Model file for the job. Use its own axes, mm. A direction names the side the tool comes from. Coordinates: 2 decimals unless noted, no trailing zeros. Write each loop counter-clockwise with the first axis right and the second up, starting at its lowest first coordinate (ties: lowest second). Pieces come first, ordered by that corner, then holes. Notation, with made-up numbers: M -37,-32.5 L -23,-32.5 A28 cw -23,-4.5 Z; hole C -26,47 d9. An arc over 180 degrees is marked long. Answer in a Markdown table with one row per item. Add a question column.
```python
from build123d import *

# Parameters (mm, degrees)
SKETCH_1_W          = 26
SKETCH_1_H          = 23.5
SKETCH_1_W_2        = 24
SKETCH_1_H_2        = 21.5
EXTRUDE_1_DEPTH     = 10
SKETCH_2_W          = 12.504676962
SKETCH_2_H          = 3.66933463
CUT_EXTRUDE_1_DEPTH = 1
EXTRUDE_2_DEPTH     = 2.3
SKETCH_5_W          = 26
SKETCH_5_H          = 23.5
EXTRUDE_3_DEPTH     = 1
CUT_EXTRUDE_2_REACH = 38.168
SKETCH_6_W          = 24.2
SKETCH_6_H          = 21.7
SKETCH_6_W_2        = 24
SKETCH_6_H_2        = 21.5
SKETCH_7_W          = 22.2
SKETCH_7_H          = 1
SKETCH_7_W_2        = 1
SKETCH_7_H_2        = 19.7
SKETCH_7_W_3        = 6.19724131
SKETCH_7_H_3        = 1.03
SKETCH_7_W_4        = 6.2
EXTRUDE_4_DEPTH     = 5.75
FILLET_1_R          = 0.95


with BuildPart() as part:
    # 草图1 → 凸台-拉伸1 (new body)
    with BuildSketch(Plane(origin=(0, 0, 0), x_dir=(1, 0, 0), z_dir=(0, 1, 0))):
        with Locations((12, 10.75)):
            Rectangle(SKETCH_1_W, SKETCH_1_H)
        with Locations((12, 10.75)):
            Rectangle(SKETCH_1_W_2, SKETCH_1_H_2, mode=Mode.SUBTRACT)
    extrude(amount=EXTRUDE_1_DEPTH)

    # 草图2 → 切除-拉伸1 (cut)
    with BuildSketch(Plane.ZY.offset(1)):
        with Locations((-10.334237592, 1.834667315)):
            Rectangle(SKETCH_2_W, SKETCH_2_H)
    extrude(amount=-CUT_EXTRUDE_1_DEPTH, mode=Mode.SUBTRACT)

    # 草图3 → 凸台-拉伸2 (add)
    with BuildSketch(Plane.XZ):
        Polygon((-1, -4.081899111), (-1, 1), (25, 1), (25, -22.5), (-1, -22.5), (-1, -16.586576073), (0, -16.586576073), (0, -21.5), (24, -21.5), (24, 0), (0, 0), (0, -4.081899111), align=None)
    extrude(amount=EXTRUDE_2_DEPTH)

    # 草图5 → 凸台-拉伸3 (add)
    with BuildSketch(Plane.XZ.offset(2.3)):
        with Locations((12, -10.75)):
            Rectangle(SKETCH_5_W, SKETCH_5_H)
    extrude(amount=EXTRUDE_3_DEPTH)

    # 切除-拉伸2: up to this face of the body (flat: up to its plane)
    cut_extrude_2_end = Plane(part.part.faces().sort_by_distance((11.704243938, -2.3, -10.74016286))[0])
    # 草图6 → 切除-拉伸2 (cut, up to the picked face)
    with BuildSketch(Plane(origin=(0, 10, 0), x_dir=(1, 0, 0), z_dir=(0, 1, 0)), mode=Mode.PRIVATE) as cut_extrude_2_sk1:
        with Locations((12, 10.75)):
            Rectangle(SKETCH_6_W, SKETCH_6_H)
        with Locations((12, 10.75)):
            Rectangle(SKETCH_6_W_2, SKETCH_6_H_2, mode=Mode.SUBTRACT)
    cut_extrude_2_tool1 = split(extrude(cut_extrude_2_sk1.sketch, amount=-CUT_EXTRUDE_2_REACH, mode=Mode.PRIVATE), bisect_by=cut_extrude_2_end, keep=Keep.BOTH, mode=Mode.PRIVATE)
    add(cut_extrude_2_tool1.solids().sort_by(Axis((12, 10, -21.567496), (0, -1, 0)))[0], mode=Mode.SUBTRACT)

    # 草图7 → 凸台-拉伸4 (add)
    with BuildSketch(Plane(origin=(0, -2.3, 0), x_dir=(1, 0, 0), z_dir=(0, 1, 0))):
        with Locations((12, 21.1)):
            Rectangle(SKETCH_7_W, SKETCH_7_H)
        with Locations((0.4, 21.1)):
            Rectangle(SKETCH_7_W_2, SKETCH_7_H)
        Polygon((0.9, 20.6), (-0.1, 20.6), (-0.1, 16.8), (0.9, 16.8), (0.9, 17.83), align=None)
        with Locations((23.6, 21.1)):
            Rectangle(SKETCH_7_W_2, SKETCH_7_H)
        with Locations((23.6, 10.75)):
            Rectangle(SKETCH_7_W_2, SKETCH_7_H_2)
        with Locations((12, 0.4)):
            Rectangle(SKETCH_7_W, SKETCH_7_H)
        with Locations((23.6, 0.4)):
            Rectangle(SKETCH_7_W_2, SKETCH_7_H)
        with Locations((0.4, 0.4)):
            Rectangle(SKETCH_7_W_2, SKETCH_7_H)
        Polygon((-0.1, 0.9), (0.9, 0.9), (0.9, 3.081899111), (0.9, 4.081899111), (-0.1, 4.081899111), align=None)
        with Locations((3.998620655, 17.315)):
            Rectangle(SKETCH_7_W_3, SKETCH_7_H_3)
        with Locations((4, 3.581899111)):
            Rectangle(SKETCH_7_W_4, SKETCH_7_H)
    extrude(amount=EXTRUDE_4_DEPTH)

    # 圆角1
    fillet_1_edges = [part.edges().sort_by_distance(p)[0] for p in [
        (-0.1, 6.725, 0.1),
        (24.1, 6.725, 0.1),
        (24.1, 6.725, -21.6),
        (-0.1, 6.725, -21.6),
        (-1, 3.35, -22.5),
        (25, 3.35, -22.5),
        (25, 3.35, 1),
        (-1, 3.35, 1),
    ]]
    fillet(fillet_1_edges, radius=FILLET_1_R)


solid = part.part
```
1) Slice it at A-A (z = -12). Give the cut face in (x, y), then the cut area to 3 significant figures.
2) Drill centre lines: probe 1 along Z at (x, y) = (3.5, -0.25); probe 2 along X at (y, z) = (2, -1.5); probe 3 along X at (y, z) = (8.5, -12.5). Where is each one in solid material? Low to high.
3) Which spindle directions (+Z, -Z, +X, -X, +Y, -Y) get a long thin tool onto all of the face, cutting with end or side? Do faces 1 (the face through (4, 1, -3.082)), 2 (the face through (-0.6, 0.6, -16.587)), 3 (the face through (12, 3, 1)). Say none if no direction does.
4) Two-plate mould, pull along Z, no slides. Class faces 4 (the face through (7.097, 1, -17)), 5 (the face through (11, 10, 0.5)), 6 (the face through (12, 3, -22.5)): released by +Z, released by -Z, zero draft, split by the parting line, or undercut.
5) Flat gauge pins, fed straight in: pin 1 Ø10 at (x, z) = (11, -8) entering from +Y; pin 2 Ø8 at (x, z) = (22, -3) entering from +Y. Where does each tip first touch, or does it go through?
6) Slice it at B-B (y = 7). Give the cut face in (x, z), then the cut area to 3 significant figures.
7) Slice it at C-C (x = 4.5). Give the cut face in (y, z).
8) Slice it at D-D (z = -19.25). Give the cut face in (x, y).
Ans:
| question | item | result |
|---|---|---|
| 1 | outline | M -1,-3.3 L 25,-3.3 L 25,10 L 24.1,10 L 24.1,3.45 L 23.1,3.45 L 23.1,-2.3 L -1,-2.3 Z; M -1,3.67 L -0.1,3.67 L -0.1,10 L -1,10 Z |
| 1 | area | 48.5 mm2 |
| 2 | probe 1 | z = -22.5 to -20.6, -17.83 to -16.8, -4.08 to -3.08, -0.9 to 1 |
| 2 | probe 2 | x = -1 to 0.9, 23.1 to 25 |
| 2 | probe 3 | x = -1 to -0.1, 24.1 to 25 |
| 3 | face 1 | +Y |
| 3 | face 2 | -X |
| 3 | face 3 | +Z, +X, -X, +Y, -Y |
| 4 | face 4 | undercut |
| 4 | face 5 | zero draft |
| 4 | face 6 | released by -Z |
| 5 | pin 1 | stops at y = -2.3 |
| 5 | pin 2 | stops at y = 10 |
| 6 | outline | M -1,-21.55 A0.95 ccw -0.05,-22.5 L 24.05,-22.5 A0.95 ccw 25,-21.55 L 25,0.05 A0.95 ccw 24.05,1 L -0.05,1 A0.95 ccw -1,0.05 Z; hole M -0.1,-20.65 A0.95 ccw 0.85,-21.6 L 23.15,-21.6 A0.95 ccw 24.1,-20.65 L 24.1,-0.85 A0.95 ccw 23.15,0.1 L 0.85,0.1 A0.95 ccw -0.1,-0.85 Z |
| 6 | area | 85.9 mm2 |
| 7 | outline | M -3.3,-22.5 L 10,-22.5 L 10,-21.6 L 3.45,-21.6 L 3.45,-20.6 L -2.3,-20.6 L -2.3,-17.83 L 3.45,-17.83 L 3.45,-16.8 L -2.3,-16.8 L -2.3,-4.08 L 3.45,-4.08 L 3.45,-3.08 L -2.3,-3.08 L -2.3,-0.9 L 3.45,-0.9 L 3.45,0.1 L 10,0.1 L 10,1 L -3.3,1 Z |
| 8 | outline | M -1,-3.3 L 25,-3.3 L 25,10 L 24.1,10 L 24.1,3.45 L 23.1,3.45 L 23.1,-2.3 L 0.9,-2.3 L 0.9,3.45 L -0.1,3.45 L -0.1,10 L -1,10 Z |
